from build123d import *

# Parameters (mm, degrees)
SKETCH_1_R          = 41.275
EXTRUDE_1_DEPTH     = 5
SKETCH_5_R          = 13
EXTRUDE_5_DEPTH     = 42
CHAMFER_3_SIZE      = 2
FILLET_1_R          = 2
EXTRUDE_START       = -0.630683
EXTRUDE_7_DEPTH     = 2.630683
CHAMFER_4_SIZE      = 0.5
SKETCH_11_R         = 65.391227149
CUT_EXTRUDE_1_DEPTH = 5


with BuildPart() as part:
    # 草图1 → 凸台-拉伸1 (new body)
    with BuildSketch(Plane.XY):
        Circle(SKETCH_1_R)
    extrude(amount=EXTRUDE_1_DEPTH)

    # 草图5 → 凸台-拉伸5 (add)
    with BuildSketch(Plane(origin=(0, 0, 0), x_dir=(-1, 0, 0), z_dir=(0, 0, -1))):
        Circle(SKETCH_5_R)
    extrude(amount=EXTRUDE_5_DEPTH)

    # 倒角3
    chamfer_3_edges = [part.edges().sort_by_distance(p)[0] for p in [
        (13, 0, -42),
    ]]
    chamfer(chamfer_3_edges, length=CHAMFER_3_SIZE)

    # 圆角1
    fillet_1_edges = [part.edges().sort_by_distance(p)[0] for p in [
        (13, 0, 0),
    ]]
    fillet(fillet_1_edges, radius=FILLET_1_R)

    # 草图10 → 凸台-拉伸7 (add)
    with BuildSketch(Plane(origin=(0, 13, 0), x_dir=(-1, 0, 0), z_dir=(0, 1, 0)).offset(EXTRUDE_START)):
        with BuildLine():
            Line((-4, -9), (-4, -33))
            ThreePointArc((-4, -33), (0, -37), (4, -33))
            Line((4, -33), (4, -9))
            ThreePointArc((4, -9), (0, -5), (-4, -9))
        make_face()
    extrude(amount=EXTRUDE_7_DEPTH)

    # 倒角4
    chamfer_4_edges = [part.edges().sort_by_distance(p)[0] for p in [
        (0, 15, -37),
        (-4, 15, -21),
        (0, 15, -5),
        (4, 15, -21),
    ]]
    chamfer(chamfer_4_edges, length=CHAMFER_4_SIZE)

    # 草图11 → 切除-拉伸1 (cut)
    with BuildSketch(Plane.XY.offset(5)):
        Circle(SKETCH_11_R)
    extrude(amount=-CUT_EXTRUDE_1_DEPTH, mode=Mode.SUBTRACT)


solid = part.part
Model file for the job. Use its own axes, mm. A direction names the side the tool comes from. Give positions to 0.01 mm unless a question says otherwise; leave off trailing zeros. Loops run counter-clockwise (first coordinate to the right, second up) from the corner with the lowest first, then second, coordinate; pieces in that order, holes last.
Item 1: Drill centre lines: line 1 along X through (y, z) = (13, -16); line 2 along Z through (x, y) = (5.25, -11.75); line 3 along X through (y, z) = (10.25, -5). Where is each one in solid material? Low to high.
Check values:
line 1: x = -4 to 4
line 2: z = -40.13 to 0
line 3: x = -8 to 8
Item 2: Slice it at A-A (x = 0). Write the cut outline in (y, z).
Check values:
outline: (-15, 0) arc R2 cw to (-13, -2) - (-13, -40) - (-11, -42) - (11, -42) - (13, -40) - (13, -37) - (14.5, -37) - (15, -36.5) - (15, -5.5) - (14.5, -5) - (13, -5) - (13, -2) arc R2 cw to (15, 0) - close
Item 3: Drop flat-ended pins along their axis: P1, Ø2, axis at x = 7.5, z = -24.5, coming from the -Y side; P2, Ø1.1, axis at y = 13.5, z = -21, coming from the +X side; P3, Ø5, axis at x = 11.5, z = -33.5, coming from the -Y side. Give the stop position or say it passes through.
Check values:
P1: stops at y = -11.26
P2: stops at x = 4
P3: stops at y = -9.38
Item 4: Slice it at C-C (y = 0). Write the cut outline in (x, z).
Check values:
outline: (-15, 0) arc R2 cw to (-13, -2) - (-13, -40) - (-11, -42) - (11, -42) - (13, -40) - (13, -2) arc R2 cw to (15, 0) - close
Item 5: Slice it at B-B (z = -19). Write the cut outline in (x, y).
Check values:
outline: (-4, 12.37) arc R13 ccw (long way) to (4, 12.37) - (4, 14.5) - (3.5, 15) - (-3.5, 15) - (-4, 14.5) - close
Item 6: Which spindle directions (+Z, -Z, +X, -X, +Y, -Y) get a long thin tool onto all of the face, cutting with end or side? Do faces 1 (the face through (-0.08, 14.865, -5.365)), 2 (the face through (0, 14, -37)), 3 (the face through (-4, 13, -21)). Say none if no direction does.
Check values:
face 1: +Y
face 2: -Z, +Y
face 3: -Z, -X, +Y
